CAD build for the part. Positions are in the model's coordinates, mm. Give positions to 0.01 mm unless a question says otherwise; leave off trailing zeros. Loops run counter-clockwise (first coordinate to the right, second up) from the corner with the lowest first, then second, coordinate; pieces in that order, holes last.
```python
from build123d import *

# Parameters (mm, degrees)
EXTRUDE1_DEPTH  = 12.8
HOLE_WIZARD_D_D = 12.3


with BuildPart() as part:
    # Sketch1 → Extrude1 (new body)
    with BuildSketch(Plane(origin=(0, 0, 0), x_dir=(1, 0, 0), z_dir=(0, 1, 0))):
        Polygon((5.5, 9.526279442), (-5.5, 9.526279442), (-11, 0), (-5.5, -9.526279442), (5.5, -9.526279442), (11, 0), align=None)
    extrude(amount=EXTRUDE1_DEPTH)

    # d (through all)
    with Locations(Plane(origin=(0, 12.8, 0), x_dir=(-1, 0, 0), z_dir=(0, 1, 0))):
        with Locations((0, 0)):
            Hole(HOLE_WIZARD_D_D / 2)

    # Sketch5 → Cut-Revolve1 (revolve, cut)
    with BuildSketch(Plane(origin=(0, 0, 0), x_dir=(0, 0, -1), z_dir=(1, 0, 0))):
        Polygon((-9.526279442, 12.8), (-11.5, 11.660471904), (-11.5, 12.8), align=None)
        Polygon((-11.5, 0), (-9.526279442, 0), (-11.5, 1.139528096), align=None)
    revolve(axis=Axis((0, 0, 0), (0, 1, 0)), mode=Mode.SUBTRACT)

    # Sketch7 → Cut-Revolve2 (revolve, cut)
    with BuildSketch(Plane(origin=(0, 0, 0), x_dir=(0, 0, -1), z_dir=(1, 0, 0)), mode=Mode.PRIVATE) as cut_revolve2_sk:
        Polygon((-7, 12.8), (-6.15, 12.8), (-6.15, 11.95), align=None)
        Polygon((-6.15, 0.85), (-7, 0), (-6.15, 0), align=None)
    revolve(cut_revolve2_sk.sketch.rotate(Axis((0, 0, 0), (0, 1, 0)), 180), axis=Axis((0, 0, 0), (0, 1, 0)), mode=Mode.SUBTRACT)


solid = part.part
```
1. Pull direction X, two halves, no side cores. Call faces 1 (the face through (-4.921, 12.593, -8.572)), 2 (the face through (-6, 12.8, -4)), 3 (the face through (4.921, 12.593, 8.572)), 4 (the face through (5.68, 6.32, -2.36)): released by +X, released by -X, zero draft, split by the parting line, or undercut.
Responses:
face 1: released by -X
face 2: zero draft
face 3: released by +X
face 4: undercut
2. Saw through at A-A, the plane y = 5.75. List the corners of the cut face in (x, z), and give its area (3 significant figures).
Responses:
outline: (-11, 0) - (-5.5, -9.53) - (5.5, -9.53) - (11, 0) - (5.5, 9.53) - (-5.5, 9.53) - close; hole circle Ø12.3 at (0, 0)
area: 196 mm2
3. Drop flat-ended pins along their axis: pin 1 (4 mm diameter, centred on x = -6.5, y = 11, fed in from +Z); pin 2 (5 mm diameter, centred on y = 2.5, z = 3, fed in from -X); pin 3 (3 mm diameter, centred on y = 4.5, z = 5, fed in from -X); pin 4 (1 mm diameter, centred on y = 4.5, z = 5, fed in from -X). Give the stop position or say it passes through.
Responses:
pin 1: stops at z = 9.53
pin 2: stops at x = -10.71
pin 3: stops at x = -8.98
pin 4: stops at x = -8.4
4. Probe line 1 along Z through (x, y) = (2.75, 3.75); line 2 along Z through (x, y) = (-1.5, 1.75); line 3 along X through (y, z) = (4, 2.5). List the from-to ranges inside material, lowest first.
Responses:
line 1: z = -9.53 to -5.5, 5.5 to 9.53
line 2: z = -9.53 to -5.96, 5.96 to 9.53
line 3: x = -9.56 to -5.62, 5.62 to 9.56
